Check sheet for the drawn part. Datum: minimum x, y, z corner. Units: mm. Round coordinates to 2 decimals unless told otherwise and drop trailing zeros. Order: outer loops, then holes, each group sorted by start corner. A loop starts at its lowest first (then second) coordinate and runs counter-clockwise, first axis right, second up.
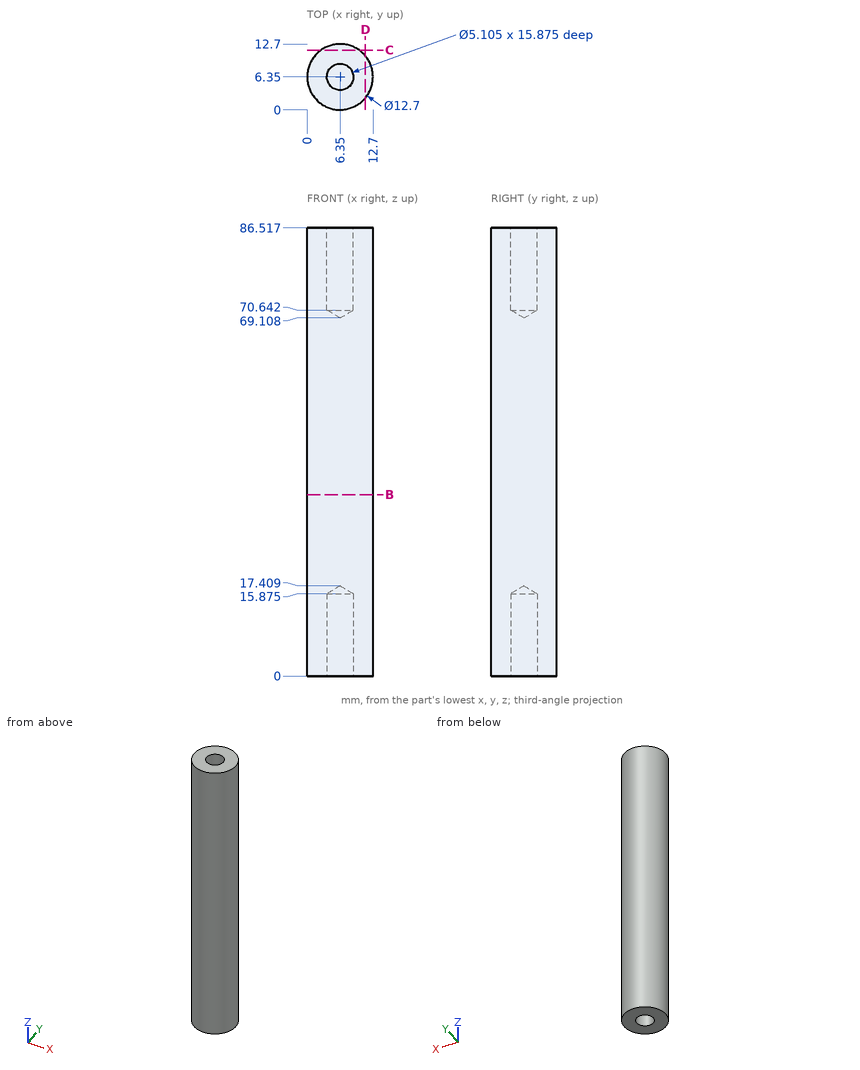
(1) Material ranges on line 1 (Y direction, x = 6.35, z = 12.5); line 2 (X direction, y = 7.5, z = 7) (1 decimal), recorded low to high.
Returned:
line 1: y = 0 to 3.8, 8.9 to 12.7
line 2: x = 0.1 to 4.1, 8.6 to 12.6
(2) Sectioned sample at C-C, the plane y = 11.5. Record the cut outline in (x, z) (1 decimal).
Returned:
outline: (2.6, 0) - (10.1, 0) - (10.1, 86.5) - (2.6, 86.5) - close
(3) Sectioned sample at B-B, the plane z = 35. Record the cut outline in (x, y), and give its area (3 significant figures).
Returned:
outline: circle Ø12.7 at (6.35, 6.35)
area: 127 mm2
(4) Sectioned sample at D-D, the plane x = 11.25. Record the cut outline in (y, z), and give its area (3 significant figures).
Returned:
outline: (2.31, 0) - (10.39, 0) - (10.39, 86.52) - (2.31, 86.52) - close
area: 699 mm2
(5) Depth check by flat-ended pin: P1, Ø4, axis at x = 6.35, y = 6.35, coming from the +Z side; P2, Ø1, axis at y = 1.5, z = 76, coming from the +X side (1 decimal); P3, Ø1.5, axis at y = 5, z = 57.5, coming from the -X side. Enter the tip coordinate at first touch or a pass-through.
Returned:
P1: stops at z = 70.31
P2: stops at x = 11
P3: stops at x = 0.03
